For this review, take the finished solid that the model builds, in its own axes (mm). A direction names the side the tool comes from. Give positions to 0.01 mm unless a question says otherwise; leave off trailing zeros. Order: outer loops, then holes, each group sorted by start corner. A loop starts at its lowest first (then second) coordinate and runs counter-clockwise, first axis right, second up.
Item 1: For probe 1 along X at (y, z) = (-1.75, -14); probe 2 along Z at (x, y) = (14, -1.5); probe 3 along Z at (x, y) = (-11.5, -5), list the stretches that pass through material, from the lowest coordinate up.
Item 2: For P1, Ø6, axis at x = 38, y = -5, coming from the +Z side; P2, Ø6.5, axis at x = -5.5, y = -6, coming from the -Z side; P3, Ø1.5, axis at y = -2, z = -8, coming from the +X side, all flat-tipped, find the tip position at first contact; note any pin that passes through.
Item 3: Machinability: for faces 1 (the flat face through (8.57, -6.44, 24.41)), 2 (the flat face through (3, 0, 0)), which of the approach directions +Z, -Z, +X, -X, +Y, -Y give a long, thin tool a straight path to every point of the face, cutting with its end or side? Answer none if there is none.
Item 4: Consider section D-D (z = -42). Give the boundary of the cut face in (x, y).
Item 5: Consider section C-C (x = -35.5). Give the boundary of the cut face in (y, z), plus the area to 3 significant figures.
Item 6: Consider section A-A (y = -8.5). Give the boundary of the cut face in (x, z) (3 decimals), plus the area to 3 significant figures.
Item 7: The part is to be moulded in two halves that separate along Z. For faces 3 (the cylindrical face through (46.704, -6.261, 14.708)), 4 (the flat face through (3, -12.7, 0)), 5 (the flat face through (-1, -6, 5.272)), say which applies: released by +Z, released by -Z, zero draft, split by the parting line, or undercut.
Item 8: Consider section B-B (z = 7). Give the boundary of the cut face in (x, y), plus the area to 3 significant figures.
```python
from build123d import *

# Parameters (mm, degrees)
F0_R     = 48.9649925961
F1_DEPTH = 12.7
F2_R     = 43.5622333877
F3_DEPTH = 12.7
F5_DEPTH = 12.7


with BuildPart() as f1:
    # F0 (on Front) → F1 (new body)
    with BuildSketch(Plane.XZ):
        Circle(F0_R)
    extrude(amount=F1_DEPTH)

    # F2 (on face) → F3 (cut)
    with BuildSketch(Plane.XZ.offset(12.7)):
        Circle(F2_R)
    extrude(amount=-F3_DEPTH, mode=Mode.SUBTRACT)

    # F4 (on face) → F5 (join)
    with BuildSketch(Plane.XZ.offset(12.7)):
        with BuildLine():
            ThreePointArc((17.379015252, 39.9454378696), (16.8725994385, 40.1619666589), (16.363486545, 40.3720755698))
            Line((16.363486545, 40.3720755698), (-7.7529065311, 5.2719768137))
            Line((-7.7529065311, 5.2719768137), (5.271977745, 5.2719768137))
            Line((5.271977745, 5.2719768137), (-8.9933723211, -13.0248842761))
            Line((-8.9933723211, -13.0248842761), (4.3416288681, -13.0248842761))
            Line((4.3416288681, -13.0248842761), (-17.2422079718, -40.004680251))
            ThreePointArc((-17.2422079718, -40.004680251), (-16.6644241691, -40.2487906009), (-16.0831855031, -40.4845565839))
            Line((-16.0831855031, -40.4845565839), (11.4743020386, -10.1048769623))
            Line((11.4743020386, -10.1048769623), (0, -10.1048769623))
            Line((0, -10.1048769623), (13.334998861, 9.3034887686))
            Line((13.334998861, 9.3034887686), (0, 9.3034887686))
            Line((0, 9.3034887686), (17.379015252, 39.9454378696))
        make_face()
    extrude(amount=-F5_DEPTH)


solid = f1.part
```
Resolved:
1. probe 1: x = -46.92 to -41.25, 3.56 to 7.94, 41.25 to 46.92
1. probe 2: z = -46.92 to -41.25, 33.99 to 36.93, 41.25 to 46.92
1. probe 3: z = -47.6 to -42.02, -35.43 to -32.83, 42.02 to 47.6
2. P1: stops at z = 34.24
2. P2: stops at z = -48.91
2. P3: stops at x = 48.43
3. face 1: +Y, -Y
3. face 2: +Z, -Z, +X, -X, +Y
4. outline: (-25.17, -12.7) - (-11.56, -12.7) - (-11.56, 0) - (-25.17, 0) - close; (11.56, -12.7) - (25.17, -12.7) - (25.17, 0) - (11.56, 0) - close
5. outline: (-12.7, -33.72) - (0, -33.72) - (0, -25.25) - (-12.7, -25.25) - close; (-12.7, 25.25) - (0, 25.25) - (0, 33.72) - (-12.7, 33.72) - close
5. area: 215 mm2
6. outline: circle Ø97.93 at (0, 0); hole (-17.242, -40.005) - (4.342, -13.025) - (-8.993, -13.025) - (5.272, 5.272) - (-7.753, 5.272) - (16.363, 40.372) arc R43.562 ccw to start; hole (-16.083, -40.485) arc R43.562 ccw to (17.379, 39.945) - (0, 9.303) - (13.335, 9.303) - (0, -10.105) - (11.474, -10.105) - close
6. area: 1,970 mm2
7. face 3: split by the parting line
7. face 4: zero draft
7. face 5: undercut
8. outline: (-48.46, -12.7) - (-43, -12.7) - (-43, 0) - (-48.46, 0) - close; (-6.57, -12.7) - (11.75, -12.7) - (11.75, 0) - (-6.57, 0) - close; (43, -12.7) - (48.46, -12.7) - (48.46, 0) - (43, 0) - close
8. area: 371 mm2
